from build123d import *

# Parameters (mm, degrees)
BOSS_EXTRU_1_DEPTH      = 2.1
ESQUISSE3_W             = 2.74226184
ESQUISSE3_H             = 0.472482842
ENL_V_MAT_EXTRU_1_DEPTH = 2.1
ESQUISSE5_R             = 0.25
BOSS_EXTRU_2_DEPTH      = 34


with BuildPart() as part:
    # Esquisse1 → Boss.-Extru.1 (new body)
    with BuildSketch(Plane(origin=(0, 0, 0), x_dir=(1, 0, 0), z_dir=(0, 1, 0))):
        with BuildLine():
            Line((-1.37113092, -2.15), (1.37113092, -2.15))
            ThreePointArc((1.37113092, -2.15), (2.55, 0), (1.37113092, 2.15))
            Line((1.37113092, 2.15), (-1.37113092, 2.15))
            ThreePointArc((-1.37113092, 2.15), (-2.55, 0), (-1.37113092, -2.15))
        make_face()
    extrude(amount=BOSS_EXTRU_1_DEPTH)

    # Esquisse2 → Révolution1 (revolve)
    with BuildSketch(Plane.XY):
        with BuildLine():
            Line((0, 2.1), (0, 2.25))
            ThreePointArc((0, 2.25), (-1.277203977, 2.212467617), (-2.55, 2.1))
            Line((-2.55, 2.1), (0, 2.1))
        make_face()
    revolve(axis=Axis((0, 2.1, 0), (0, 1, 0)))

    # Esquisse3 → Enlèv. mat.-Extru.1 (cut)
    with BuildSketch(Plane.XZ.offset(-2.1)):
        with Locations((0, -2.386241421)):
            Rectangle(ESQUISSE3_W, ESQUISSE3_H)
        Polygon((-1.37113092, 2.15), (-1.37113092, 2.636321801), (1.307781681, 2.636321801), (1.37113092, 2.15), align=None)
    extrude(amount=-ENL_V_MAT_EXTRU_1_DEPTH, mode=Mode.SUBTRACT)

    # Esquisse5 → Boss.-Extru.2 (add)
    with BuildSketch(Plane(origin=(0, 2.25, 0), x_dir=(1, 0, 0), z_dir=(0, 1, 0))):
        with Locations(Location((-1.5, 0, 0), (0, 0, 270))):
            Circle(ESQUISSE5_R)
        with Locations(Location((1.5, 0, 0), (0, 0, 270))):
            Circle(ESQUISSE5_R)
    extrude(amount=-BOSS_EXTRU_2_DEPTH)


solid = part.part
Verification items for the finished model (mm, model axes). Round coordinates to 2 decimals unless told otherwise and drop trailing zeros. Order: outer loops, then holes, each group sorted by start corner. A loop starts at its lowest first (then second) coordinate and runs counter-clockwise, first axis right, second up. Notation, with made-up numbers: (34, -21) -> (51, -21) arc R23 cw to (51, -12) -> close; hole circle Ø4 at (-3, 20). An arc over 180 degrees is marked (long way). Put each result on its own line as item: value.
1) Section check C-C (z = -1.55). Record the cut outline in (x, y).
Final values:
outline: (-2.02, 0) -> (2.02, 0) -> (2.02, 2.1) arc R21.69 ccw to (-2.02, 2.1) -> close
2) Section check B-B (x = -2.15). Record the cut outline in (y, z).
Final values:
outline: (0, -1.37) -> (2.1, -1.37) arc R21.64 ccw to (2.1, 1.37) -> (0, 1.37) -> close
3) Material ranges on line 1 (X direction, y = -25, z = -0.05); line 2 (Y direction, x = -1.65, z = -1.35); line 3 (Y direction, x = -1.1, z = 1.2), recorded low to high.
Final values:
line 1: x = -1.74 to -1.26, 1.26 to 1.74
line 2: y = 0 to 2.15
line 3: y = 0 to 2.19
4) Section check A-A (y = -11.5). Record the cut outline in (x, z), then the cut area to 3 significant figures.
Final values:
outline: circle Ø0.5 at (-1.5, 0); circle Ø0.5 at (1.5, 0)
area: 0.393 mm^2
5) Depth check by flat-ended pin: pin 1 (1.5 mm diameter, centred on y = -27.5, z = 0, fed in from +X); pin 2 (1.5 mm diameter, centred on x = -1, y = -17, fed in from -Z); pin 3 (2 mm diameter, centred on x = -0.5, z = 1.5, fed in from +Y); pin 4 (2 mm diameter, centred on x = 1, z = 0, fed in from -Y). Enter the tip coordinate at first touch or a pass-through.
Final values:
pin 1: stops at x = 1.75
pin 2: stops at z = -0.25
pin 3: stops at y = 2.24
pin 4: stops at y = -31.75
